The listing builds one solid part. Answer for the finished solid, in the listing's coordinates (mm). Give positions to 0.01 mm unless a question says otherwise; leave off trailing zeros. Loops run counter-clockwise (first coordinate to the right, second up) from the corner with the lowest first, then second, coordinate; pieces in that order, holes last. Notation, with made-up numbers: (48, 44) - (101, 44) arc R16 ccw to (101, 67) - close; hole circle Ø10 at (42, 71). An arc over 180 degrees is marked (long way). Answer in a Markdown table with one row per item. Add a question column.
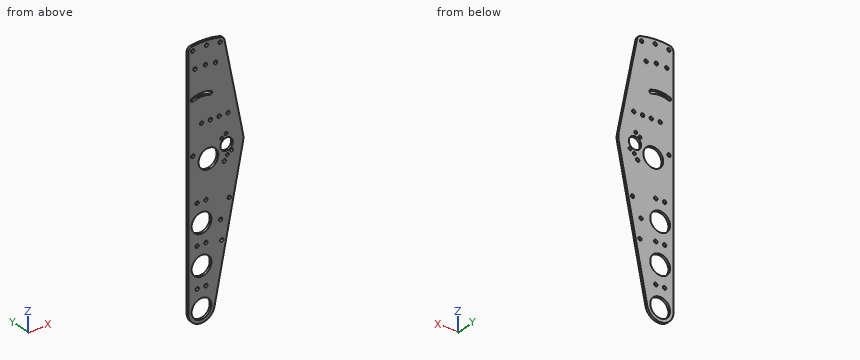
Autodesk Inventor part; units mm, degrees
ref_plane "YZ Plane" through (0, 0, 0) normal (1, 0, 0) x (0, 1, 0)
ref_plane "XZ Plane" through (0, 0, 0) normal (0, 1, 0) x (-1, 0, 0)
ref_plane "XY Plane" through (0, 0, 0) normal (0, 0, 1) x (1, 0, 0)
sketch "Sketch1" plane through (0, 0, 0) normal (0, 1, 0) x (-1, 0, 0)
  circle A0 centre (0, 0) radius 2.4892
  arc A1 (13.031, 35.8023) -> (-13.031, 35.8023) centre (0, 0) ccw construction
  arc A2 (13.904, 38.201) -> (-13.904, 38.201) centre (0, 0) ccw
  arc A3 (12.1579, 33.4035) -> (-12.1579, 33.4035) centre (0, 0) ccw
  arc A4 (12.1579, 33.4035) -> (13.904, 38.201) centre (13.031, 35.8023) ccw
  arc A5 (-13.904, 38.201) -> (-12.1579, 33.4035) centre (-13.031, 35.8023) ccw
  circle A6 centre (9.525, 75.6023) radius 2.4892
  circle A7 centre (12.7, 100.8031) radius 2.4892
  circle A8 centre (6.35, -218.4769) radius 2.4892
  circle A9 centre (-5.4073, 76.0079) radius 2.4892
  circle A10 centre (-20.1318, 73.4925) radius 2.4892
  line L0 (0, 0) -> (12.7, 100.8031) construction
  circle A11 centre (-7.2097, 101.3439) radius 2.4892
  circle A12 centre (-26.8424, 97.99) radius 2.4892
  line L1 (-7.2097, 101.3439) -> (0, 0) construction
  line L2 (0, 0) -> (0, 59.2895) construction
  line L3 (13.031, 35.8023) -> (0, 0) construction
  line L4 (-13.031, 35.8023) -> (0, 0) construction
  circle A13 centre (0, -247.0519) radius 14.2875
  line L5 (19.05, -247.0519) -> (19.05, 100.8031)
  arc A14 (19.05, 100.8031) -> (13.4937, 107.1033) centre (12.7, 100.8031) ccw
  arc A15 (-28.5201, 104.1144) -> (-33.0721, 99.2201) centre (-26.8424, 97.99) ccw
  arc A16 (13.4937, 107.1033) -> (-28.5201, 104.1144) centre (0, 0) ccw
  line L6 (0, 0) -> (-40.6527, 0) construction
  circle A17 centre (-6.35, -218.4769) radius 2.4892
  circle A18 centre (6.35, -161.3269) radius 2.4892
  circle A19 centre (-6.35, -161.3269) radius 2.4892
  circle A20 centre (6.35, -104.1769) radius 2.4892
  circle A21 centre (-6.35, -104.1769) radius 2.4892
  circle A22 centre (0, -189.9019) radius 14.2875
  circle A23 centre (0, -132.7519) radius 14.2875
  line L7 (0, -247.0519) -> (6.35, -218.4769) construction
  line L8 (6.35, -218.4769) -> (0, -189.9019) construction
  line L9 (0, -247.0519) -> (-6.35, -218.4769) construction
  line L10 (-6.35, -218.4769) -> (0, -189.9019) construction
  line L11 (-18.6766, -250.8051) -> (-59.8526, -45.9075)
  line L12 (-59.8685, -36.4906) -> (-33.0721, 99.2201)
  circle A24 centre (-9.9191, -50.8) radius 14.2875
  circle A25 centre (-32.5382, -62.3558) radius 2.4892
  circle A26 centre (12.7, -39.2442) radius 2.4892
  circle A27 centre (-36.2243, -41.1592) radius 8.89
  circle A28 centre (-43.3377, -51.4378) radius 2.125
  circle A29 centre (-35.2937, -26.6891) radius 2.125
  circle A30 centre (-29.1109, -30.8806) radius 2.125
  circle A31 centre (-37.1549, -55.6293) radius 2.125
  arc A32 (-59.8685, -36.4906) -> (-59.8526, -45.9075) centre (-36.2243, -41.1592) ccw
  circle A33 centre (-9.9191, -50.8) radius 22.8981 construction
  circle A34 centre (-36.2243, -41.1592) radius 5.1181 construction
  circle A35 centre (-37.1549, -55.6293) radius 4.7625 construction
  circle A36 centre (-29.1109, -30.8806) radius 4.7625 construction
  line L13 (0, -247.0519) -> (0, -189.9019) construction
  line L14 (16.3478, -247.0519) -> (16.3478, -189.9019) construction
  line L15 (-16.3478, -189.9019) -> (-16.3478, -247.0519) construction
  arc A37 (-16.3478, -247.0519) -> (16.3478, -247.0519) centre (0, -247.0519) ccw construction
  arc A38 (16.3478, -189.9019) -> (-16.3478, -189.9019) centre (0, -189.9019) ccw construction
  line L16 (0, -189.9019) -> (0, -132.7519) construction
  line L17 (17.8104, -189.9019) -> (17.8104, -132.7519) construction
  line L18 (-17.8104, -132.7519) -> (-17.8104, -189.9019) construction
  arc A39 (-17.8104, -189.9019) -> (17.8104, -189.9019) centre (0, -189.9019) ccw construction
  arc A40 (17.8104, -132.7519) -> (-17.8104, -132.7519) centre (0, -132.7519) ccw construction
  line L19 (0, -132.7519) -> (-9.9191, -50.8) construction
  line L20 (-17.6814, -134.892) -> (-27.6005, -52.9401) construction
  line L21 (7.7622, -48.6599) -> (17.6814, -130.6118) construction
  arc A41 (-17.6814, -134.892) -> (17.6814, -130.6118) centre (0, -132.7519) ccw construction
  arc A42 (7.7622, -48.6599) -> (-27.6005, -52.9401) centre (-9.9191, -50.8) ccw construction
  line L22 (-32.5382, -62.3558) -> (12.7, -39.2442) construction
  line L23 (-60.325, -8.1201) -> (-60.325, -77.446) construction
  circle A43 centre (-12.7, 0) radius 2.4892
  circle A44 centre (-25.4, 0) radius 2.4892
  circle A45 centre (-38.1, 0) radius 2.4892
  circle A46 centre (-38.1, 0) radius 14.2875 construction
  line L24 (19.05, -12.7) -> (-50.1557, -12.7) construction
  line L25 (-50.1557, -12.7) -> (-50.1557, 12.7) construction
  line L26 (-50.1557, 12.7) -> (19.05, 12.7) construction
  line L27 (19.05, 12.7) -> (19.05, -12.7) construction
  line L28 (19.05, -12.7) -> (-50.1557, 12.7) construction
  line L29 (-50.1557, -12.7) -> (19.05, 12.7) construction
  arc A47 (-18.6766, -250.8051) -> (19.05, -247.0519) centre (0, -247.0519) ccw
  circle A48 centre (12.7, -39.2442) radius 6.35 construction
  circle A49 centre (-29.2174, -166.1224) radius 2.4892
  circle A50 centre (-39.8407, -113.2593) radius 6.35 construction
  circle A51 centre (-27.381, -138.2544) radius 2.4892
  line L30 (-29.2174, -166.1224) -> (-27.381, -138.2544) construction
  line L31 (-27.381, -138.2544) -> (-39.8407, -113.2593) construction
  circle A52 centre (-29.2174, -166.1224) radius 6.35 construction
  circle A53 centre (-39.8407, -113.2593) radius 2.4892
  line L32 (0, -132.7519) -> (-27.381, -138.2544) construction
  circle A54 centre (-27.381, -138.2544) radius 13.6409 construction
  circle A55 centre (0, -247.0519) radius 50.8 construction
  circle A56 centre (0, -132.7519) radius 50.8 construction
  line L33 (-33.8517, -66.4129) -> (0.3232, -77.4763) construction
  line L34 (5.6938, -74.7325) -> (16.7572, -40.5577) construction
  line L35 (14.0134, -35.1871) -> (-20.1614, -24.1237) construction
  line L36 (-25.5321, -26.8675) -> (-36.5954, -61.0423) construction
  line L37 (-37.9089, -65.0995) -> (18.0706, -36.5005) construction
  line L38 (4.3804, -78.7897) -> (-24.2186, -22.8103) construction
  arc A57 (-36.5954, -61.0423) -> (-33.8517, -66.4129) centre (-32.5382, -62.3558) ccw construction
  arc A58 (16.7572, -40.5577) -> (14.0134, -35.1871) centre (12.7, -39.2442) ccw construction
  arc A59 (-20.1614, -24.1237) -> (-25.5321, -26.8675) centre (-21.4749, -28.1809) ccw construction
  arc A60 (0.3232, -77.4763) -> (5.6938, -74.7325) centre (1.6366, -73.4191) ccw construction
  circle A61 centre (-32.5382, -62.3558) radius 6.0334 construction
  point P0 (0, -218.4769)
  point P1 (0, -161.3269)
  point P2 (-4.9596, -91.7759)
  point P3 (-15.5529, 0)
  dimension "d0" = 4.9784
  dimension "d1" = 38.1
  dimension "d2" = 5.1054
  dimension "d5" = 22.5
  dimension "d7" = 14.9378
  dimension "d8" = 25.4
  dimension "d11" = 22.5
  dimension "d13" = 76.2
  dimension "d14" = 40
  dimension "d15" = 28.575
  dimension "d18" = 12.7
  dimension "d19" = 107.95
  dimension "d22" = 12.7
  dimension "d25" = 57.15
  dimension "d30" = 57.15
  dimension "d35" = 28.575
  dimension "d38" = 360
  dimension "d40" = 50.8
  dimension "d41" = 17.78
  dimension "d44" = 360
  dimension "d46" = 29
  dimension "d48" = 4.25
  dimension "d49" = 25
  dimension "d50" = 45.7962
  dimension "d51" = 10.2362
  dimension "d52" = 82.55
  dimension "d54" = 297.062
  dimension "d55" = 50.8
  dimension "d56" = 9.525
  dimension "d57" = 79.375
  dimension "d60" = 12.7
  dimension "d66" = 28.575
  dimension "d67" = 25.4
  dimension "d68" = 4.7625
  dimension "d70" = 12.7
  dimension "d72" = 35.6208
  dimension "d75" = 101.6
  dimension "d76" = 101.6
  dimension "d77" = 44.45
  dimension "d78" = 4.2645
extrude "Extrusion1" add sketch "Sketch1" along normal blind 3.175
equation "\"d30\" = d25"
properties part number "GreyT Claw Top V2" material "Aluminum 6061"
(1) A cutting plane is placed at A-A on y = 0.7. Give the number of separate pieces and of enclosed holes in the cut face, plus the area to 3 significant figures.
(2) A cutting plane is placed at B-B on z = 52. Determine the outline of the cut face in (x, y) (3 decimals), plus the area to 3 significant figures.
(3) Given pin 1 Ø4.5 at (x, z) = (25.4, 0) entering from -Y, flat-ended and moving along its own axis, determine where the tip first touches the part or whether it passes through.
(4) Find the intervals of material crossed by line 1 along X through (y, z) = (3, -48); line 2 along X through (y, z) = (2.35, -39); line 3 along X through (y, z) = (1.15, -135), in increasing order. Write a range as [from, to].
Evaluation:
| question | item | result |
|---|---|---|
| 1 | separate pieces | 1 |
| 1 | enclosed holes | 31 |
| 1 | area | 19,000 mm² |
| 2 | outline | (-19.05, 0) - (42.396, 0) - (42.396, 3.175) - (-19.05, 3.175) - close |
| 2 | area | 195 mm² |
| 3 | pin 1 | passes through |
| 4 | line 1 | x = [-19.05, -4.09], [23.93, 30.55], [41.9, 59.43] |
| 4 | line 2 | x = [-19.05, -15.18], [-10.22, 1.86], [17.97, 27.6], [44.85, 60.23] |
| 4 | line 3 | x = [-19.05, -14.11], [14.11, 41.95] |
